Could you check a few things on this model? Use its own coordinates, in mm. Face numbers are marked on the shaded views. A direction names the side the tool comes from. Coordinates: 2 decimals unless noted, no trailing zeros. Loops run counter-clockwise (first coordinate to the right, second up) from the corner with the lowest first, then second, coordinate; pieces in that order, holes last. Notation, with made-up numbers: (23, -8.75) - (42, -8.75) arc R26 ccw to (42, 13.25) - close; hole circle Ø3 at (26.5, 7). An arc over 180 degrees is marked (long way). One line per item, written item: value. Start each with the question number.
(1) On a 3-axis mill with a long thin cutter (end or side, diameter ignored), from which of +Z, -Z, +X, -X, +Y, -Y can I reach the whole of each face in a straight line? I mean the marked faces 1, 2, 3, 4 and 5. Say none if no direction works.
(2) If we section it at B-B on x = 18: Write out the boundary of the cut face in (y, z), then the cut area to 3 significant figures.
(3) If we section it at D-D on z = 41.5: Write out the boundary of the cut face in (x, y), then the cut area to 3 significant figures.
(4) If I drill on line 1 along X through (y, z) = (10, 28); line 2 along X through (y, z) = (-25, 4); line 3 along X through (y, z) = (23, -0.5), over which ranges is the centre line in solid material (lowest first)? Write a range as from..to.
(5) I'm going to push flat-ended pins straight in: P1, Ø12, axis at x = 121.5, y = 24, coming from the -Z side; P2, Ø8, axis at x = 41, z = -5, coming from the +Y side (3 decimals); P3, Ø1, axis at x = 117.5, z = 26, coming from the -Y side. Where does each tip first touch, or does it pass through?
(6) If we mould it in two halves opening along X, with no side actions, what happens to the marked faces 6, 7, 8 and 9? For each: pulls with the +X half, pulls with the -X half, needs draft (parallel to the pull), parting line crosses it, or undercut.
(7) If we section it at C-C on z = 30: Count the separate pieces of the cut face and the enclosed holes in it, then the cut area to 3 significant figures.
(8) If we section it at A-A on y = -42: Write out the boundary of the cut face in (x, z), then the cut area to 3 significant figures.
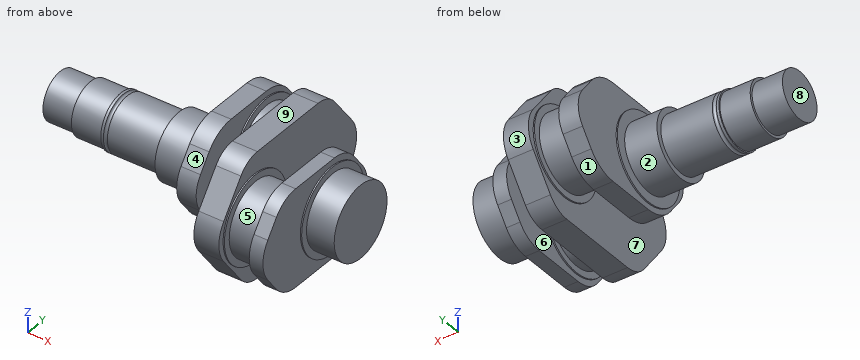
Autodesk Inventor part; units mm, degrees
ref_plane "Work Plane7" through (130.26, 0, 0) normal (1, 0, 0) x (0, 0, -1)
ref_plane "Work Plane8" through (172.17, 34.5, 0) normal (1, 0, 0) x (0, 0, -1)
ref_plane "YZ Plane" through (0, 0, 0) normal (1, 0, 0) x (0, 1, 0)
sketch "Sketch1" plane through (0, 0, 0) normal (0, 0, 1) x (1, 0, 0)
  line L0 (0, 0) -> (115.5, 0)
  line L1 (0, 0) -> (0, 18)
  line L2 (0, 18) -> (23, 18)
  line L3 (23, 18) -> (23, 20)
  line L4 (23, 20) -> (46, 20)
  line L5 (46, 20) -> (46, 21)
  line L6 (46, 21) -> (48, 21)
  arc A0 (48, 21) -> (51, 21) centre (49.5, 21) ccw
  line L7 (51, 21) -> (90, 21)
  line L8 (90, 21) -> (90, 25)
  line L9 (115.5, 32.5) -> (115.5, 0)
  line L10 (90, 25) -> (114.5, 25)
  line L11 (114.5, 25) -> (114.5, 32.5)
  line L12 (114.5, 32.5) -> (115.5, 32.5)
  dimension "d1" = 23
  dimension "d2" = 23
  dimension "d3" = 44
  dimension "d4" = 36
  dimension "d6" = 40
  dimension "d7" = 42
  dimension "d9" = 25.5
  dimension "d10" = 2
  dimension "d11" = 1.5
  dimension "d13" = 65
  dimension "d14" = 50
  dimension "d15" = 1
revolve "Revolution1" add sketch "Sketch1" angle 360 about axis through (0, 0, 0) along (1, 0, 0)
ref_plane "Work Plane7" through (130.26, 0, 0) normal (1, 0, 0) x (0, 0, -1)
sketch "Sketch22" plane through (130.26, 0, 0) normal (1, 0, 0) x (0, 0, -1)
  circle A0 centre (0, 34.5) radius 32.5
  circle A1 centre (0, 34.5) radius 27.5
  point P0 (0, 0)
  dimension "d97" = 65
  dimension "d98" = 55
  dimension "d99" = 34.5
extrude "Extrusion18" add sketch "Sketch22" along normal blind 22 contours A1
extrude "Extrusion19" add sketch "Sketch22" along normal blind 1
sketch "Sketch23" plane through (115.5, 0, 0) normal (1, 0, 0) x (0, 0, -1)
  line L0 (-37, -1.125) -> (-37, 35.625)
  line L1 (37, -1.125) -> (37, 35.625)
  arc A0 (-37, -1.125) -> (-25.6, -23.925) centre (-8.5, -1.125) ccw
  arc A1 (25.6, -23.925) -> (37, -1.125) centre (8.5, -1.125) ccw
  line L2 (-25.6, -23.925) -> (-13.6, -32.925)
  line L3 (25.6, -23.925) -> (13.6, -32.925)
  arc A2 (-13.6, -32.925) -> (13.6, -32.925) centre (0, -14.7917) ccw
  line L4 (4.9524, -36.9107) -> (32.7905, -16.0321) construction
  circle A3 centre (0, 0) radius 32.5
  line L5 (-37, 17.25) -> (37, 17.25) construction
  arc A4 (-25.6, 58.425) -> (-37, 35.625) centre (-8.5, 35.625) ccw
  arc A5 (37, 35.625) -> (25.6, 58.425) centre (8.5, 35.625) ccw
  line L6 (-25.6, 58.425) -> (-13.6, 67.425)
  line L7 (25.6, 58.425) -> (13.6, 67.425)
  arc A6 (13.6, 67.425) -> (-13.6, 67.425) centre (0, 49.2917) ccw
  line L8 (4.9524, 71.4107) -> (32.7905, 50.5321) construction
  circle A7 centre (0, 34.5) radius 32.5 construction
  dimension "d105" = 15
  dimension "d106" = 74
  dimension "d107" = 27.2
  dimension "d108" = 51.2
  dimension "d109" = 2
  dimension "d126" = 2
extrude "Extrusion20" add sketch "Sketch23" along normal up to surface (14.76 mm away) contours L0 A4 L6 A6 L7 A5 L1 A1 L3 A2 L2 A0 | A3
sketch "Sketch24" plane through (152.26, 34.5, 0) normal (1, 0, 0) x (0, 0, -1)
  circle A0 centre (0, 0) radius 32.5
  point P0 (0, -34.5)
extrude "Extrusion21" add sketch "Sketch24" along normal blind 1
ref_plane "Work Plane8" through (172.17, 34.5, 0) normal (1, 0, 0) x (0, 0, -1)
sketch "Sketch25" plane through (172.17, 34.5, 0) normal (1, 0, 0) x (0, 0, -1)
  circle A0 centre (0, -69) radius 32.5
  circle A1 centre (0, 0) radius 32.5 construction
  point P0 (0, -34.5)
  dimension "d115" = 65
  dimension "d116" = 69
extrude "Extrusion22" add sketch "Sketch25" along normal blind 1
sketch "Sketch26" plane through (153.26, 34.5, 0) normal (1, 0, 0) x (0, 0, -1)
  arc A0 (15, 32.4583) -> (-15, 32.4583) centre (0, 12.4583) ccw
  line L0 (-15, 32.4583) -> (-38.92, 14.5183)
  line L1 (15, 32.4583) -> (38.92, 14.5183)
  arc A1 (47.5, -2.6417) -> (38.92, 14.5183) centre (26.05, -2.6417) ccw
  arc A2 (-38.92, 14.5183) -> (-47.5, -2.6417) centre (-26.05, -2.6417) ccw
  line L2 (-47.5, -2.6417) -> (-47.5, -65.775)
  line L3 (47.5, -2.6417) -> (47.5, -65.775)
  arc A3 (13.6, 32.925) -> (-13.6, 32.925) centre (0, 14.7917) ccw
  line L4 (-47.5, -34.2083) -> (47.5, -34.2083) construction
  line L5 (13.6, 32.925) -> (25.6, 23.925)
  arc A4 (-15, -100.875) -> (15, -100.875) centre (0, -80.875) ccw
  line L6 (-15, -100.875) -> (-38.92, -82.935)
  line L7 (15, -100.875) -> (38.92, -82.935)
  arc A5 (38.92, -82.935) -> (47.5, -65.775) centre (26.05, -65.775) ccw
  arc A6 (-47.5, -65.775) -> (-38.92, -82.935) centre (-26.05, -65.775) ccw
  line L8 (5.9616, -105.1538) -> (30.4845, -86.7616) construction
  circle A7 centre (0, -69) radius 32.5
  point P0 (0, -34.5)
  point P1 (0, 37.4583)
  dimension "d119" = 25
  dimension "d120" = 29.9
  dimension "d122" = 95
  dimension "d127" = 2
extrude "Extrusion23" add sketch "Sketch26" along normal up to surface (18.91 mm away) contours L1 A1 L3 A5 L7 A4 L6 A6 L2 A2 L0 A0 | A7
sketch "Sketch27" plane through (173.17, -34.5, 0) normal (1, 0, 0) x (0, 0, -1)
  circle A0 centre (0, 0) radius 27.5
  circle A1 centre (0, 0) radius 32.5
  point P0 (0, 34.5)
  dimension "d128" = 55
extrude "Extrusion24" add sketch "Sketch27" along normal blind 21 contours A0
sketch "Sketch28" plane through (194.17, -34.5, 0) normal (1, 0, 0) x (0, 0, -1)
  circle A0 centre (0, 0) radius 32.5
  point P0 (0, 34.5)
extrude "Extrusion25" add sketch "Sketch28" along normal blind 1
sketch "Sketch29" plane through (195.17, -34.5, 0) normal (1, 0, 0) x (0, 0, -1)
  arc A0 (-15, -31.875) -> (15, -31.875) centre (0, -11.875) ccw
  line L0 (-15, -31.875) -> (-27, -22.875)
  line L1 (38.92, -13.935) -> (15, -31.875) construction
  line L2 (15, -31.875) -> (27, -22.875)
  line L3 (-15, -31.875) -> (-38.92, -13.935) construction
  arc A1 (27, -22.875) -> (37, -2.875) centre (12, -2.875) ccw
  arc A2 (-37, -2.875) -> (-27, -22.875) centre (-12, -2.875) ccw
  line L4 (-37, -2.875) -> (-37, 37.525)
  line L5 (37, -2.875) -> (37, 37.525)
  arc A3 (-27, 57.525) -> (-37, 37.525) centre (-12, 37.525) ccw
  arc A4 (37, 37.525) -> (27, 57.525) centre (12, 37.525) ccw
  line L6 (-27, 57.525) -> (-15, 66.525)
  line L7 (27, 57.525) -> (15, 66.525)
  arc A5 (15, 66.525) -> (-15, 66.525) centre (0, 46.525) ccw
  point P0 (0, 34.5)
  dimension "d133" = 15
  dimension "d134" = 25
  dimension "d135" = 40.4
  dimension "d136" = 25
extrude "Extrusion26" add sketch "Sketch29" along normal blind 10.43
sketch "Sketch30" plane through (205.6, -34.5, 0) normal (1, 0, 0) x (0, 0, -1)
  circle A0 centre (0, 34.5) radius 18 construction
  circle A1 centre (0, 34.5) radius 32.5
  dimension "d139" = 65
extrude "Extrusion27" add sketch "Sketch30" along normal blind 1
sketch "Sketch31" plane through (206.6, 0, 0) normal (1, 0, 0) x (0, 0, -1)
  circle A0 centre (0, 0) radius 27.5
  dimension "d142" = 55
extrude "Extrusion28" add sketch "Sketch31" along normal blind 21
ref_plane "Work Plane9" through (217.1, 0, 0) normal (1, 0, 0) x (0, 0, -1)
properties part number "Korbowód poprawiony"
Values:
1. face 1: -Z, -X, +Y
1. face 2: -X
1. face 3: +X, -X, +Y
1. face 4: +Z, -X, -Y
1. face 5: none
2. outline: circle Ø36 at (0, 0)
2. area: 1,020 mm2
3. outline: (153.26, -46.15) - (172.17, -46.15) - (172.17, 46.74) - (153.26, 46.74) - close
3. area: 1,760 mm2
4. line 1: x = 114.5..130.26, 153.26..172.17, 195.17..206.6
4. line 2: x = 114.5..130.26, 153.26..227.6
4. line 3: x = 90..172.17, 195.17..227.6
5. P1: stops at z = -37
5. P2: stops at y = 19.975
5. P3: stops at y = -24
6. face 6: undercut
6. face 7: undercut
6. face 8: pulls with the -X half
6. face 9: needs draft
7. separate pieces: 3
7. enclosed holes: 0
7. area: 4,120 mm2
8. outline: (153.26, -44.63) - (172.17, -44.63) - (172.17, -31.62) - (173.17, -31.62) - (173.17, -26.46) - (194.17, -26.46) - (194.17, -31.62) - (195.17, -31.62) - (195.17, -36.57) - (205.6, -36.57) - (205.6, 36.57) - (195.17, 36.57) - (195.17, 31.62) - (194.17, 31.62) - (194.17, 26.46) - (173.17, 26.46) - (173.17, 31.62) - (172.17, 31.62) - (172.17, 44.63) - (153.26, 44.63) - close
8. area: 3,690 mm2
